For this review, use the dimensioned drawing (mm, ordinates from the lowest corner) and the shaded views. A direction names the side the tool comes from. Coordinates: 2 decimals unless noted, no trailing zeros. Order: outer loops, then holes, each group sorted by start corner. A loop starts at its lowest first (then second) coordinate and runs counter-clockwise, first axis right, second up. Notation, with made-up numbers: M 42.5,86 L 49.5,86 A18 ccw 49.5,90 Z; hole C 27,67 d1. An arc over 180 degrees is marked long. One line per item, written item: value.
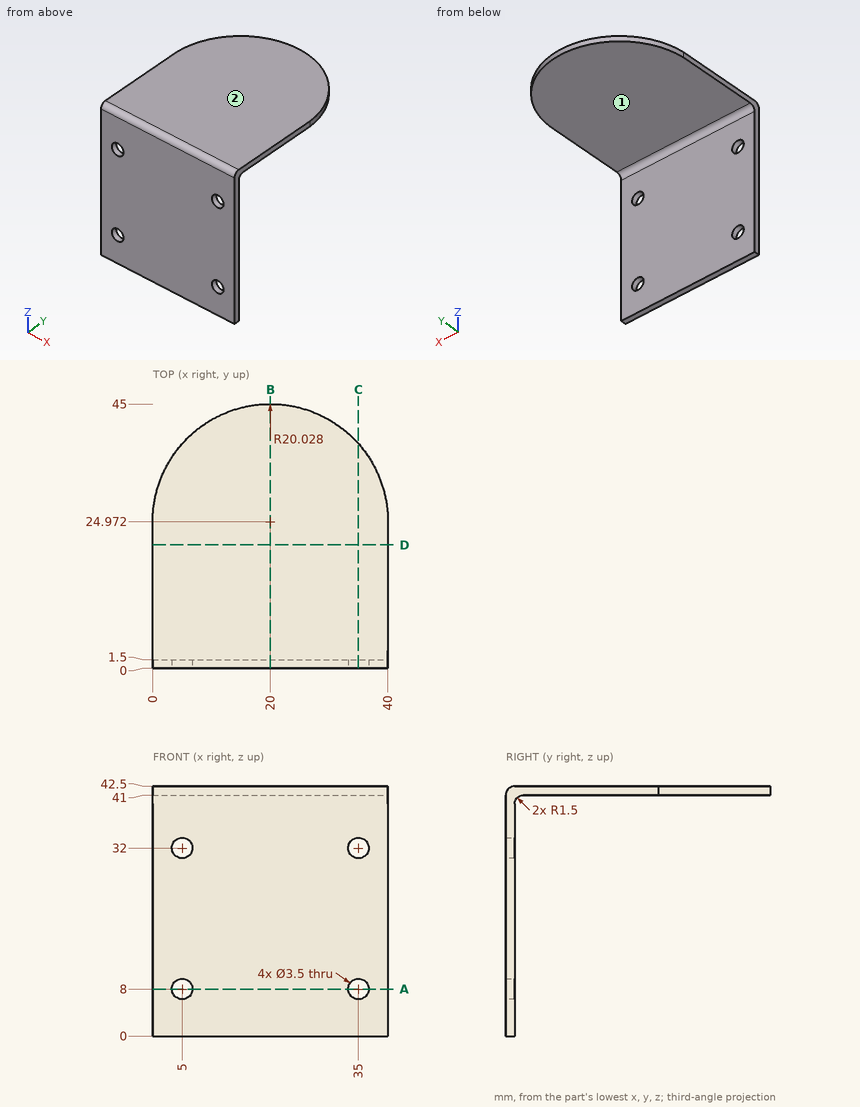
(1) For L1, parallel to X at y = 0.65, z = 32; L2, parallel to Y at x = 18, z = 30; L3, parallel to Z at x = 3.5, y = 22, list the stretches that pass through material, from the lowest coordinate up.
Geometry results:
L1: x = 0 to 3.25, 6.75 to 33.25, 36.75 to 40
L2: y = 0 to 1.5
L3: z = 41 to 42.5
(2) Tool access review of the marked faces 1 and 2: name each direction out of +Z, -Z, +X, -X, +Y, -Y from which nothing blocks a thin tool from reaching the whole face with its end or side.
Geometry results:
face 1: -Z, +X, -X, +Y
face 2: +Z, +X, -X, +Y, -Y
(3) Insertion check: pin 1 Ø4 at (x, z) = (5, 8) entering from +Y; pin 2 Ø10 at (y, z) = (32, 37) entering from -X; pin 3 Ø12 at (x, y) = (19.5, 22) entering from -Z. Each pin has a flat end and moves straight along its axis. Give the tip position at first contact, or say it passes through.
Geometry results:
pin 1: stops at y = 1.5
pin 2: stops at x = 0.38
pin 3: stops at z = 41
(4) We need section D-D, the plane y = 21. State the section outline as (x, z) points.
Geometry results:
outline: M 0,41 L 40,41 L 40,42.5 L 0,42.5 Z
(5) We need section C-C, the plane x = 35. State the section outline as (y, z) points, plus the area to 3 significant figures.
Geometry results:
outline: M 0,0 L 1.5,0 L 1.5,6.25 L 0,6.25 Z; M 0,9.75 L 1.5,9.75 L 1.5,30.25 L 0,30.25 Z; M 0,33.75 L 1.5,33.75 L 1.5,39.5 A1.5 cw 3,41 L 38.24,41 L 38.24,42.5 L 1.5,42.5 A1.5 ccw 0,41 Z
area: 108 mm2
(6) We need section B-B, the plane x = 20. State the section outline as (y, z) points.
Geometry results:
outline: M 0,0 L 1.5,0 L 1.5,39.5 A1.5 cw 3,41 L 45,41 L 45,42.5 L 1.5,42.5 A1.5 ccw 0,41 Z
(7) We need section A-A, the plane z = 8. State the section outline as (x, y) points.
Geometry results:
outline: M 0,0 L 3.25,0 L 3.25,1.5 L 0,1.5 Z; M 6.75,0 L 33.25,0 L 33.25,1.5 L 6.75,1.5 Z; M 36.75,0 L 40,0 L 40,1.5 L 36.75,1.5 Z
